The model under review builds one solid part; all positions refer to its coordinate system, in mm. A direction names the side the tool comes from. Coordinates: 2 decimals unless noted, no trailing zeros. Loops run counter-clockwise (first coordinate to the right, second up) from the corner with the lowest first, then second, coordinate; pieces in that order, holes last. Notation, with made-up numbers: (14.5, 24) - (53.5, 24) arc R8 cw to (53.5, 34) - close; hole circle Ø9 at (74, 78.5). An arc over 180 degrees is marked (long way). One line per item, written item: value. Start each with the question number.
1. For faces 4 (the face through (3.3, 0.1, 11)), 5 (the face through (5.25, 0.03, 10.01)), 6 (the face through (5, -2, 9)), list the 3-axis set-ups (+Z, -Z, +X, -X, +Y, -Y) from which the entire face can be reached by the end or side of a thin tool; tool diameter is ignored.
2. We need section B-B, the plane z = 10.5. Give the boundary of the cut face in (x, y), then the cut area to 3 significant figures.
3. Mouldability with a two-part tool opening along X and no side actions: class faces 1 (the face through (-1.5, 5.26, 3.43)), 2 (the face through (5, -2, 7)), 3 (the face through (-1.73, -7.81, 9.99)) as +X half, -X half, draft (parallel to the pull), parting line (faces both ways), or undercut.
4. We need section D-D, the plane y = 5.75. Count the separate pieces of the cut face and the enclosed holes in it, then the cut area to 3 significant figures.
5. Insertion check: P1, Ø2, axis at y = 3.5, z = 3.5, coming from the +X side; P2, Ø4.5, axis at x = 0.5, y = 2, coming from the +Z side; P3, Ø2, axis at y = 3.5, z = 7.5, coming from the +X side; P4, Ø0.9, axis at x = 6, y = 0, coming from the +Z side. Each pin has a flat end and moves straight along its axis. Give the tip position at first contact, or say it passes through.
6. To check wall thickness, follow line 1 (Z direction, x = 0, y = 6.3); line 2 (Z direction, x = 4.5, y = -5.25); line 3 (Z direction, x = 1.25, y = 6.5). State the ranges of each line that lie inside material, in increasing order.
7. We need section A-A, the plane y = 0. Give the boundary of the cut face in (x, z), then the cut area to 3 significant figures.
8. We need section C-C, the plane z = 5.75. Give the boundary of the cut face in (x, y).
from build123d import *

# Parameters (mm, degrees)
SKETCH1_R           = 8
BOSS_EXTRUDE1_DEPTH = 11
SKETCH2_W           = 2
SKETCH2_H           = 3
CUT_EXTRUDE1_REACH  = 12.5
CUT_EXTRUDE1_START  = 2.5
SKETCH5_R           = 1.5
CUT_EXTRUDE2_REACH  = 13
SKETCH6_R           = 3
FILLET3_R           = 0.25
FILLET4_R           = 0.25
FILLET5_R           = 0.25
CUT_EXTRUDE3_REACH  = 13
SKETCH7_R           = 0.75


with BuildPart() as part:
    # Sketch1 → Boss-Extrude1 (new body)
    with BuildSketch(Plane.XY):
        Circle(SKETCH1_R)
    extrude(amount=BOSS_EXTRUDE1_DEPTH)

    # Sketch2 → Cut-Revolve2 (revolve, cut)
    with BuildSketch(Plane(origin=(0, 0, 0), x_dir=(0, 0, -1), z_dir=(1, 0, 0))):
        with Locations((-8, 6.5)):
            Rectangle(SKETCH2_W, SKETCH2_H)
    revolve(axis=Axis((0, 0, -5.249485175), (0, 0, 1)), mode=Mode.SUBTRACT)

    # Sketch5 → Cut-Extrude1 (cut, up to next)
    with BuildSketch(Plane(origin=(0, 0, 0), x_dir=(1, 0, 0), z_dir=(0, 1, 0)).offset(CUT_EXTRUDE1_START), mode=Mode.PRIVATE) as cut_extrude1_sk1:
        with Locations((0, -3.5)):
            Circle(SKETCH5_R)
    cut_extrude1_tool1 = extrude(cut_extrude1_sk1.sketch, amount=CUT_EXTRUDE1_REACH, mode=Mode.PRIVATE) & part.part
    add(cut_extrude1_tool1.solids().sort_by_distance((0, 2.5, 3.5))[0], mode=Mode.SUBTRACT)

    # Sketch6 → Cut-Extrude2 (cut, up to next)
    with BuildSketch(Plane.XY, mode=Mode.PRIVATE) as cut_extrude2_sk1:
        Circle(SKETCH6_R)
    cut_extrude2_tool1 = extrude(cut_extrude2_sk1.sketch, amount=CUT_EXTRUDE2_REACH, mode=Mode.PRIVATE) & part.part
    add(cut_extrude2_tool1.solids().sort_by_distance((0, 0, 0))[0], mode=Mode.SUBTRACT)

    # Fillet3
    fillet3_edges = [part.edges().sort_by_distance(p)[0] for p in [
        (-8, 0, 9),
    ]]
    fillet(fillet3_edges, radius=FILLET3_R)

    # Fillet4
    fillet4_edges = [part.edges().sort_by_distance(p)[0] for p in [
        (-8, 0, 7),
    ]]
    fillet(fillet4_edges, radius=FILLET4_R)

    # Fillet5
    fillet5_edges = [part.edges().sort_by_distance(p)[0] for p in [
        (-8, 0, 0),
        (-8, 0, 11),
    ]]
    fillet(fillet5_edges, radius=FILLET5_R)

    # Sketch7 → Cut-Extrude3 (cut, up to next)
    with BuildSketch(Plane.XY.offset(11), mode=Mode.PRIVATE) as cut_extrude3_sk1:
        with Locations((6, 0)):
            Circle(SKETCH7_R)
    cut_extrude3_tool1 = extrude(cut_extrude3_sk1.sketch, amount=-CUT_EXTRUDE3_REACH, mode=Mode.PRIVATE) & part.part
    add(cut_extrude3_tool1.solids().sort_by_distance((6, 0, 11))[0], mode=Mode.SUBTRACT)


solid = part.part
Findings below:
1. face 4: +Z, +X, -X, +Y, -Y
1. face 5: +Z
1. face 6: none
2. outline: circle Ø16 at (0, 0); hole circle Ø6 at (0, 0); hole circle Ø1.5 at (6, 0)
2. area: 171 mm2
3. face 1: undercut
3. face 2: draft
3. face 3: parting line
4. separate pieces: 2
4. enclosed holes: 1
4. area: 92.9 mm2
5. P1: x = 7.6
5. P2: z = 11
5. P3: x = 7.5
5. P4: z = 7
6. line 1: 0 to 2, 5 to 7, 9 to 11
6. line 2: 0 to 7, 9 to 11
6. line 3: 0 to 2.67, 4.33 to 7, 9 to 11
7. outline: (-8, 0.25) arc R0.25 ccw to (-7.75, 0) - (-3, 0) - (-3, 11) - (-7.75, 11) arc R0.25 ccw to (-8, 10.75) - (-8, 9.25) arc R0.25 ccw to (-7.75, 9) - (-5, 9) - (-5, 7) - (-7.75, 7) arc R0.25 ccw to (-8, 6.75) - close; (3, 0) - (7.75, 0) arc R0.25 ccw to (8, 0.25) - (8, 6.75) arc R0.25 ccw to (7.75, 7) - (5, 7) - (5, 9) - (5.25, 9) - (5.25, 11) - (3, 11) - close; (6.75, 9) - (7.75, 9) arc R0.25 ccw to (8, 9.25) - (8, 10.75) arc R0.25 ccw to (7.75, 11) - (6.75, 11) - close
7. area: 94.9 mm2
8. outline: circle Ø16 at (0, 0); hole circle Ø6 at (0, 0)
